Build history of the part. All positions in model axes, mm. A direction names the side the tool comes from. Give positions to 0.01 mm unless a question says otherwise; leave off trailing zeros. Loops run counter-clockwise (first coordinate to the right, second up) from the corner with the lowest first, then second, coordinate; pieces in that order, holes last. Notation, with made-up numbers: M 43,-16 L 79,-16 A15 cw 79,-8 Z; hole C -38,-6 d3. An arc over 180 degrees is marked long. Put each result on its own line as item: value.
```python
from build123d import *

# Parameters (mm, degrees)
BOSS_EXTRUDE2_DEPTH = 10
SKETCH2_R           = 8
CUT_EXTRUDE1_DEPTH  = 17
CUT_EXTRUDE2_DEPTH  = 20
SKETCH4_R           = 8
SKETCH4_R_2         = 2.8
BOSS_EXTRUDE3_DEPTH = 10
SKETCH5_R           = 7.78
CUT_EXTRUDE3_DEPTH  = 19


with BuildPart() as part:
    # Sketch1 → Boss-Extrude2 (new body)
    # profile 1 of 2: a face of its own
    with BuildSketch(Plane.XY):
        with BuildLine():
            ThreePointArc((-60.621778265, 45), (-56.602540378, 60), (-60.621778265, 75))
            Line((-60.621778265, 75), (-76.961524227, 103.301270189))
            Line((-76.961524227, 103.301270189), (-50.980762114, 118.301270189))
            Line((-50.980762114, 118.301270189), (-34.641016151, 90))
            ThreePointArc((-34.641016151, 90), (-23.660254038, 79.019237886), (-8.660254038, 75))
            Line((-8.660254038, 75), (8.660254038, 75))
            ThreePointArc((8.660254038, 75), (23.660254038, 79.019237886), (34.641016151, 90))
            Line((34.641016151, 90), (50.980762114, 118.301270189))
            Line((50.980762114, 118.301270189), (76.961524227, 103.301270189))
            Line((76.961524227, 103.301270189), (60.621778265, 75))
            ThreePointArc((60.621778265, 75), (56.602540378, 60), (60.621778265, 45))
            Line((60.621778265, 45), (69.282032303, 30))
            ThreePointArc((69.282032303, 30), (80.262794416, 19.019237886), (95.262794416, 15))
            Line((95.262794416, 15), (127.942286341, 15))
            Line((127.942286341, 15), (127.942286341, -15))
            Line((127.942286341, -15), (95.262794416, -15))
            ThreePointArc((95.262794416, -15), (80.262794416, -19.019237886), (69.282032303, -30))
            Line((69.282032303, -30), (60.621778265, -45))
            ThreePointArc((60.621778265, -45), (56.602540378, -60), (60.621778265, -75))
            Line((60.621778265, -75), (76.961524227, -103.301270189))
            Line((76.961524227, -103.301270189), (50.980762114, -118.301270189))
            Line((50.980762114, -118.301270189), (34.641016151, -90))
            ThreePointArc((34.641016151, -90), (23.660254038, -79.019237886), (8.660254038, -75))
            Line((8.660254038, -75), (-8.660254038, -75))
            ThreePointArc((-8.660254038, -75), (-23.660254038, -79.019237886), (-34.641016151, -90))
            Line((-34.641016151, -90), (-50.980762114, -118.301270189))
            Line((-50.980762114, -118.301270189), (-76.961524227, -103.301270189))
            Line((-76.961524227, -103.301270189), (-60.621778265, -75))
            ThreePointArc((-60.621778265, -75), (-56.602540378, -60), (-60.621778265, -45))
            Line((-60.621778265, -45), (-69.282032303, -30))
            ThreePointArc((-69.282032303, -30), (-80.262794416, -19.019237886), (-95.262794416, -15))
            Line((-95.262794416, -15), (-127.942286341, -15))
            Line((-127.942286341, -15), (-127.942286341, 15))
            Line((-127.942286341, 15), (-95.262794416, 15))
            ThreePointArc((-95.262794416, 15), (-80.262794416, 19.019237886), (-69.282032303, 30))
            Line((-69.282032303, 30), (-60.621778265, 45))
        make_face()
        Polygon((28.867513459, -50), (57.735026919, 0), (28.867513459, 50), (-28.867513459, 50), (-57.735026919, 0), (-28.867513459, -50), align=None, mode=Mode.SUBTRACT)
    # profile 2 of 2: a face of its own
    with BuildSketch(Plane.XY):
        Polygon((49.074772881, 15), (-49.074772881, 15), (-57.735026919, 0), (-49.074772881, -15), (49.074772881, -15), (57.735026919, 0), align=None)
    extrude(amount=BOSS_EXTRUDE2_DEPTH)

    # Sketch2 → Cut-Extrude1 (cut)
    with BuildSketch(Plane.XY):
        with Locations((106.241169623, 0)):
            Circle(SKETCH2_R)
        with Locations((53.120584811, -92.007551821)):
            Circle(SKETCH2_R)
        with Locations((-53.120584811, -92.007551821)):
            Circle(SKETCH2_R)
        with Locations((-106.241169623, 0)):
            Circle(SKETCH2_R)
        with Locations((-53.120584811, 92.007551821)):
            Circle(SKETCH2_R)
        with Locations((53.120584811, 92.007551821)):
            Circle(SKETCH2_R)
    extrude(amount=CUT_EXTRUDE1_DEPTH, mode=Mode.SUBTRACT)

    # Sketch3 → Cut-Extrude2 (cut)
    with BuildSketch(Plane.XY):
        Polygon((-45.669872981, -2.5), (-50, 5), (-54.330127019, -2.5), align=None)
        Polygon((-55.669872981, -2.5), (-60, 5), (-64.330127019, -2.5), align=None)
        Polygon((-35.669872981, -2.5), (-40, 5), (-44.330127019, -2.5), align=None)
        Polygon((-25.669872981, -2.5), (-30, 5), (-34.330127019, -2.5), align=None)
        Polygon((-15.669872981, -2.5), (-20, 5), (-24.330127019, -2.5), align=None)
        Polygon((-5.669872981, -2.5), (-10, 5), (-14.330127019, -2.5), align=None)
        Polygon((4.330127019, -2.5), (0, 5), (-4.330127019, -2.5), align=None)
        Polygon((14.330127019, -2.5), (10, 5), (5.669872981, -2.5), align=None)
        Polygon((24.330127019, -2.5), (20, 5), (15.669872981, -2.5), align=None)
        Polygon((34.330127019, -2.5), (30, 5), (25.669872981, -2.5), align=None)
        Polygon((44.330127019, -2.5), (40, 5), (35.669872981, -2.5), align=None)
        Polygon((54.330127019, -2.5), (50, 5), (45.669872981, -2.5), align=None)
        Polygon((64.330127019, -2.5), (60, 5), (55.669872981, -2.5), align=None)
        Polygon((-26, 60), (-33.5, 64.330127019), (-33.5, 55.669872981), align=None)
        Polygon((-35, 60), (-42.5, 64.330127019), (-42.5, 55.669872981), align=None)
        Polygon((-17, 60), (-24.5, 64.330127019), (-24.5, 55.669872981), align=None)
        Polygon((-8, 60), (-15.5, 64.330127019), (-15.5, 55.669872981), align=None)
        Polygon((1, 60), (-6.5, 64.330127019), (-6.5, 55.669872981), align=None)
        Polygon((10, 60), (2.5, 64.330127019), (2.5, 55.669872981), align=None)
        Polygon((19, 60), (11.5, 64.330127019), (11.5, 55.669872981), align=None)
        Polygon((28, 60), (20.5, 64.330127019), (20.5, 55.669872981), align=None)
        Polygon((37, 60), (29.5, 64.330127019), (29.5, 55.669872981), align=None)
        Polygon((29.5, -55.669872981), (37, -60), (29.5, -64.330127019), align=None)
        Polygon((20.5, -55.669872981), (28, -60), (20.5, -64.330127019), align=None)
        Polygon((11.5, -55.669872981), (19, -60), (11.5, -64.330127019), align=None)
        Polygon((2.5, -55.669872981), (10, -60), (2.5, -64.330127019), align=None)
        Polygon((-6.5, -55.669872981), (1, -60), (-6.5, -64.330127019), align=None)
        Polygon((-15.5, -55.669872981), (-8, -60), (-15.5, -64.330127019), align=None)
        Polygon((-24.5, -55.669872981), (-17, -60), (-24.5, -64.330127019), align=None)
        Polygon((-33.5, -55.669872981), (-26, -60), (-33.5, -64.330127019), align=None)
        Polygon((-42.5, -55.669872981), (-35, -60), (-42.5, -64.330127019), align=None)
    extrude(amount=CUT_EXTRUDE2_DEPTH, mode=Mode.SUBTRACT)

    # Sketch4 → Boss-Extrude3 (add)
    # profile 1 of 6: a face of its own
    with BuildSketch(Plane.XY):
        with Locations((106.241169623, 0)):
            Circle(SKETCH4_R)
        with Locations((106.241169623, 0)):
            Circle(SKETCH4_R_2, mode=Mode.SUBTRACT)
    # profile 2 of 6: a face of its own
    with BuildSketch(Plane.XY):
        with Locations((53.120584811, -92.007551821)):
            Circle(SKETCH4_R)
        with Locations((53.120584811, -92.007551821)):
            Circle(SKETCH4_R_2, mode=Mode.SUBTRACT)
    # profile 3 of 6: a face of its own
    with BuildSketch(Plane.XY):
        with Locations((-53.120584811, -92.007551821)):
            Circle(SKETCH4_R)
        with Locations((-53.120584811, -92.007551821)):
            Circle(SKETCH4_R_2, mode=Mode.SUBTRACT)
    # profile 4 of 6: a face of its own
    with BuildSketch(Plane.XY):
        with Locations((-106.241169623, 0)):
            Circle(SKETCH4_R)
        with Locations((-106.241169623, 0)):
            Circle(SKETCH4_R_2, mode=Mode.SUBTRACT)
    # profile 5 of 6: a face of its own
    with BuildSketch(Plane.XY):
        with Locations((-53.120584811, 92.007551821)):
            Circle(SKETCH4_R)
        with Locations((-53.120584811, 92.007551821)):
            Circle(SKETCH4_R_2, mode=Mode.SUBTRACT)
    # profile 6 of 6: a face of its own
    with BuildSketch(Plane.XY):
        with Locations((53.120584811, 92.007551821)):
            Circle(SKETCH4_R)
        with Locations((53.120584811, 92.007551821)):
            Circle(SKETCH4_R_2, mode=Mode.SUBTRACT)
    extrude(amount=BOSS_EXTRUDE3_DEPTH)

    # Sketch5 → Cut-Extrude3 (cut)
    with BuildSketch(Plane.XY):
        with Locations((106.241169623, 0)):
            Circle(SKETCH5_R)
        with Locations((53.120584811, -92.007551821)):
            Circle(SKETCH5_R)
        with Locations((-53.120584811, -92.007551821)):
            Circle(SKETCH5_R)
        with Locations((-106.241169623, 0)):
            Circle(SKETCH5_R)
        with Locations((-53.120584811, 92.007551821)):
            Circle(SKETCH5_R)
        with Locations((53.120584811, 92.007551821)):
            Circle(SKETCH5_R)
    extrude(amount=CUT_EXTRUDE3_DEPTH, mode=Mode.SUBTRACT)


solid = part.part
```
Q1. Mould opens along Y. For faces 1 (the flat face through (24.198, 57.805, 4.93)), 2 (the flat face through (64.15, -110.7, 4.93)), 3 (the flat face through (111, 15, 5)) say: pulls with the +Y half, pulls with the -Y half, needs draft (parallel to the pull), parting line crosses it, or undercut.
Here are the results:
face 1: undercut
face 2: pulls with the -Y half
face 3: pulls with the +Y half
Q2. Probe line 1 (X direction, y = -4.5, z = 6.75); line 2 (Y direction, x = 67.5, z = 6.5); line 3 (Y direction, x = -72, z = 6.5). List the from-to ranges inside material, lowest first. Write a range as from..to.
Here are the results:
line 1: -127.94..-112.59, -99.89..99.89, 112.59..127.94
line 2: -108.76..-86.91, -33.09..33.09, 86.91..108.76
line 3: -106.17..-94.71, -26.06..26.06, 94.71..106.17
Q3. Slice it at A-A (z = 8). State how many separate pieces and enclosed holes the cut face has, and give its area (3 significant figures).
Here are the results:
separate pieces: 1
enclosed holes: 39
area: 20,700 mm²
Q4. Drop flat-ended pins along their axis: pin 1 Ø6 at (y, z) = (-89, 3.5) entering from +X; pin 2 Ø4.5 at (y, z) = (-58.5, 3.5) entering from +X; pin 3 Ø2.5 at (y, z) = (59, 5.5) entering from +X. Give the stop position or say it passes through.
Here are the results:
pin 1: x = 70.44
pin 2: x = 56.84
pin 3: x = 56.69
Q5. Tool access for faces 4 (the flat face through (0, -50, 5)), 5 (the flat face through (0, -75, 5)), 6 (the flat face through (68.906, 89.349, 4.93)): list every direction of +Z, -Z, +X, -X, +Y, -Y with a clear straight run to the whole face (end or side of a thin tool).
Here are the results:
face 4: +Z, -Z
face 5: +Z, -Z, -Y
face 6: +Z, -Z, +X
Q6. Slice it at B-B (x = -92). List the corners of the cut face in (y, z), and give its area (3 significant figures).
Here are the results:
outline: M -15.18,0 L 15.18,0 L 15.18,10 L -15.18,10 Z
area: 304 mm²
Q7. Slice it at C-C (x = 81). List the corners of the cut face in (y, z).
Here are the results:
outline: M -18.61,0 L 18.61,0 L 18.61,10 L -18.61,10 Z
